from build123d import *

# Parameters (mm, degrees)
F0_R     = 9.5
F1_DEPTH = 7


with BuildPart() as f1:
    # F0 (on Top) → F1 (new body)
    with BuildSketch(Plane.XY):
        with BuildLine():
            Line((19.215132, 22.378807), (0, 55.077419))
            Line((0, 55.077419), (-19.066227, 22.201317))
            ThreePointArc((-19.066227, 22.201317), (-15.219751, 8.713844), (-28.836632, 5.354102))
            Line((-28.836632, 5.354102), (-48.016034, -27.717147))
            Line((-48.016034, -27.717147), (-9.689672, -27.717147))
            ThreePointArc((-9.689672, -27.717147), (0.044547, -17.537595), (9.778766, -27.717147))
            Line((9.778766, -27.717147), (48.653703, -27.717147))
            Line((48.653703, -27.717147), (29.068287, 5.61158))
            ThreePointArc((29.068287, 5.61158), (15.203422, 8.742665), (19.215132, 22.378807))
        make_face()
        Polygon((-23.626551, -19.414298), (-28.626551, -16.527547), (-28.626551, -10.754044), (-23.626551, -7.867293), (-18.626551, -10.754044), (-18.626551, -16.527547), align=None, mode=Mode.SUBTRACT)
        Circle(F0_R, mode=Mode.SUBTRACT)
        Polygon((28.626551, -10.754044), (28.626551, -16.527547), (23.626551, -19.414298), (18.626551, -16.527547), (18.626551, -10.754044), (23.626551, -7.867293), align=None, mode=Mode.SUBTRACT)
        Polygon((-5, 30.168342), (0, 33.055094), (5, 30.168342), (5, 24.39484), (0, 21.508088), (-5, 24.39484), align=None, mode=Mode.SUBTRACT)
    extrude(amount=F1_DEPTH)


solid = f1.part
The listing builds one solid part. Answer for the finished solid, in the listing's coordinates (mm). A direction names the side the tool comes from. Round coordinates to 2 decimals unless told otherwise and drop trailing zeros. Loops run counter-clockwise (first coordinate to the right, second up) from the corner with the lowest first, then second, coordinate; pieces in that order, holes last. Notation, with made-up numbers: M 28.25,19 L 84.25,19 A24 ccw 84.25,33 Z; hole C -18,26.5 d6. An arc over 180 degrees is marked long. Write each question's results on one line, items separated by ' | '. Start each with the question number.
1) Find section A-A on z = 5. Write down the section's boundary in (x, y).
2) Find section D-D on y = 27. Write down the section's boundary in (x, z), plus the area to 3 significant figures.
3) Straight lines are drawn through the part: probe 1 along X at (y, z) = (5, 6); probe 2 along X at (y, z) = (-19, 4.25); probe 3 along Y at (x, z) = (2, 4). For each, find the intervals that lie inside material, in ascending order.
4) Each of these flat-tipped pins is pushed along its axis until it touches: pin 1 (1.7 mm diameter, centred on y = -14.5, z = 4.5, fed in from -X); pin 2 (4 mm diameter, centred on y = -11.5, z = 4, fed in from -X); pin 3 (3 mm diameter, centred on y = -13.5, z = 3.5, fed in from +X). Where does it stop, or does it pass through?
5) Find section B-B on y = 0. Write down the section's boundary in (x, z), plus the area to 3 significant figures.
6) Which of the six approach directions +Z, -Z, +X, -X, +Y, -Y give full straight-line access (tool end or side, diameter ignored) to faces 1 (the flat face through (10, -4, 0)), 2 (the flat face through (21.09, -9.33, 3.45))?
7) Find section C-C on x = 2. Write down the section's boundary in (y, z), plus the area to 3 significant figures.
8) Determine the mould class of faces 3 (the flat face through (10, -4, 7)), 4 (the flat face through (-9.4, 38.87, 3.45)), 5 (the cylindrical face through (4.38, -8.43, 3.45)) for opening direction X: pulls with the +X half, pulls with the -X half, needs draft (parallel to the pull), parting line crosses it, or undercut.
Final values:
1) outline: M -48.02,-27.72 L -9.69,-27.72 A9.74 cw long 9.78,-27.72 L 48.65,-27.72 L 29.07,5.61 A9.74 cw long 19.22,22.38 L 0,55.08 L -19.07,22.2 A9.74 cw long -28.84,5.35 Z; hole M -28.63,-16.53 L -23.63,-19.41 L -18.63,-16.53 L -18.63,-10.75 L -23.63,-7.87 L -28.63,-10.75 Z; hole C 0,0 d19; hole M -5,24.39 L 0,21.51 L 5,24.39 L 5,30.17 L 0,33.06 L -5,30.17 Z; hole M 18.63,-16.53 L 23.63,-19.41 L 28.63,-16.53 L 28.63,-10.75 L 23.63,-7.87 L 18.63,-10.75 Z
2) outline: M -16.28,0 L -5,0 L -5,7 L -16.28,7 Z; M 5,0 L 16.5,0 L 16.5,7 L 5,7 Z | area: 159 mm²
3) probe 1: -29.04 to -28.23, -19.07 to -8.08, 8.08 to 19.18, 28.03 to 29.43 | probe 2: -42.96 to -24.34, -22.91 to -5.09, 5.18 to 22.91, 24.34 to 43.53 | probe 3: -17.74 to -9.29, 9.29 to 22.66, 31.9 to 51.67
4) pin 1: x = -40.84 | pin 2: x = -39.77 | pin 3: x = 41.18
5) outline: M -31.94,0 L -9.5,0 L -9.5,7 L -31.94,7 Z; M 9.5,0 L 32.37,0 L 32.37,7 L 9.5,7 Z | area: 317 mm²
6) face 1: -Z, +X, -X, +Y, -Y | face 2: +Z, -Z
7) outline: M -17.74,0 L -9.29,0 L -9.29,7 L -17.74,7 Z; M 9.29,0 L 22.66,0 L 22.66,7 L 9.29,7 Z; M 31.9,0 L 51.67,0 L 51.67,7 L 31.9,7 Z | area: 291 mm²
8) face 3: needs draft | face 4: pulls with the -X half | face 5: undercut
